CAD build for the part. Positions are in the model's coordinates, mm. A direction names the side the tool comes from. Round coordinates to 2 decimals unless told otherwise and drop trailing zeros. Order: outer loops, then holes, each group sorted by start corner. A loop starts at its lowest first (then second) coordinate and runs counter-clockwise, first axis right, second up.
```python
from build123d import *

# Parameters (mm, degrees)
CUT_EXTRUDE_START        = -3.5
SKETCH_4_R               = 17.25
SKETCH_4_R_2             = 16.25
CUT_EXTRUDE_1_DEPTH      = 0.5
HOLE_WIZARD_M2_5_2_D     = 2.05
HOLE_WIZARD_M2_5_2_DEPTH = 3.5
HOLE_WIZARD_M2_5_2_TIP   = 0.615882135
SKETCH_9_W               = 5.8
SKETCH_9_H               = 1.5
EXTRUDE_1_DEPTH          = 4
HOLE_WIZARD_M2_5_1_D     = 2.05
HOLE_WIZARD_M2_5_1_DEPTH = 3.5
HOLE_WIZARD_M2_5_1_TIP   = 0.615882135
FILLET_1_R               = 0.8
SKETCH_14_R              = 4
CUT_EXTRUDE_1_2_DEPTH    = 1.3


with BuildPart() as part:
    # 草图1 → 旋转1 (revolve)
    with BuildSketch(Plane.XY):
        Polygon((-6, 0), (-6, 1.62), (-17.25, 1.62), (-17.25, 16.62), (-3.25, 16.62), (-3.25, 0), align=None)
    revolve(axis=Axis((0, 44.719290515, 0), (0, -1, 0)))

    # 草图4 → Cut-Extrude 1 (cut)
    with BuildSketch(Plane.XZ.offset(-1.62).offset(CUT_EXTRUDE_START)):
        Circle(SKETCH_4_R)
        Circle(SKETCH_4_R_2, mode=Mode.SUBTRACT)
    extrude(amount=-CUT_EXTRUDE_1_DEPTH, mode=Mode.SUBTRACT)

    # M2.5 螺纹孔2
    with Locations(Plane(origin=(0, 1.62, 0), x_dir=(-1, 0, 0), z_dir=(0, -1, 0))):
        with Locations((-6.717514421, 6.717514421), (-6.717514421, -6.717514421), (6.717514421, -6.717514421), (6.717514421, 6.717514421)):
            Hole(HOLE_WIZARD_M2_5_2_D / 2, depth=HOLE_WIZARD_M2_5_2_DEPTH)
            with Locations((0, 0, -(HOLE_WIZARD_M2_5_2_DEPTH + HOLE_WIZARD_M2_5_2_TIP / 2))):  # 118° drill point
                Cone(0, HOLE_WIZARD_M2_5_2_D / 2, HOLE_WIZARD_M2_5_2_TIP, mode=Mode.SUBTRACT)

    # 草图9 → 凸台-拉伸1 (add)
    with BuildSketch(Plane.XZ.offset(-1.62)):
        with Locations((0, -14.5)):
            Rectangle(SKETCH_9_W, SKETCH_9_H)
    extrude(amount=EXTRUDE_1_DEPTH)

    # M2.5 螺纹孔1
    with Locations(Plane(origin=(0, 16.62, 0), x_dir=(1, 0, 0), z_dir=(0, 1, 0))):
        with Locations((-4.242640687, 4.242640687), (4.242640687, 4.242640687), (4.242640687, -4.242640687), (-4.242640687, -4.242640687)):
            Hole(HOLE_WIZARD_M2_5_1_D / 2, depth=HOLE_WIZARD_M2_5_1_DEPTH)
            with Locations((0, 0, -(HOLE_WIZARD_M2_5_1_DEPTH + HOLE_WIZARD_M2_5_1_TIP / 2))):  # 118° drill point
                Cone(0, HOLE_WIZARD_M2_5_1_D / 2, HOLE_WIZARD_M2_5_1_TIP, mode=Mode.SUBTRACT)

    # 圆角1
    fillet_1_edges = [part.edges().sort_by_distance(p)[0] for p in [
        (17.25, 16.62, 0),
    ]]
    fillet(fillet_1_edges, radius=FILLET_1_R)

    # 草图14 → Cut-Extrude 1 2 (cut)
    with BuildSketch(Plane.XZ):
        Circle(SKETCH_14_R)
    extrude(amount=-CUT_EXTRUDE_1_2_DEPTH, mode=Mode.SUBTRACT)


solid = part.part
```
1. Cut at A-A, the plane z = 0. Write the cut outline in (x, y).
2. Drill centre lines: line 1 (X direction, y = 13.5, z = 4); line 2 (X direction, y = 12.75, z = 0); line 3 (Z direction, x = -6.5, y = 2.5). Where is each one in solid material? Low to high.
3. Pin check, flat tips, straight feed: P1, Ø3, axis at y = 6.5, z = -7.5, coming from the -X side; P2, Ø1.2, axis at x = 4.24, z = 4.24, coming from the +Y side; P3, Ø1.6, axis at y = 0, z = -15, coming from the -X side. Stop position of each tip, or through.
4. Tool access for faces 5 (the face through (0, 0, -13.75)), 6 (the face through (-6.851, 3.394, -7.734)), 7 (the face through (-16.453, 3.394, -5.181)), 8 (the face through (-1.42, 0, 3.92)), 9 (the face through (5.267, 14.846, -4.288)): list every direction of +Z, -Z, +X, -X, +Y, -Y with a clear straight run to the whole face (end or side of a thin tool).
5. Mould opens along X. For faces 1 (the face through (2.579, 8.853, 1.978)), 2 (the face through (4.2, 12.6, 4.4)), 3 (the face through (13, 5.62, -10)), 4 (the face through (-16.453, 10.791, -5.181)) say: released by +X, released by -X, zero draft, split by the parting line, or undercut.
6. Cut at C-C, the plane y = -1. Write the cut outline in (x, z).
Outcome:
1. outline: (-17.25, 1.62) - (-6, 1.62) - (-6, 0) - (-4, 0) - (-4, 1.3) - (-3.25, 1.3) - (-3.25, 16.62) - (-16.45, 16.62) arc R0.8 ccw to (-17.25, 15.82) - (-17.25, 5.62) - (-16.25, 5.62) - (-16.25, 5.12) - (-17.25, 5.12) - close; (3.25, 1.3) - (4, 1.3) - (4, 0) - (6, 0) - (6, 1.62) - (17.25, 1.62) - (17.25, 5.12) - (16.25, 5.12) - (16.25, 5.62) - (17.25, 5.62) - (17.25, 15.82) arc R0.8 ccw to (16.45, 16.62) - (3.25, 16.62) - close
2. line 1: x = -16.78 to -5.24, -3.25 to 3.25, 5.24 to 16.78
2. line 2: x = -17.25 to -3.25, 3.25 to 17.25
2. line 3: z = -15.98 to -7.72, -5.72 to 5.72, 7.72 to 15.98
3. P1: stops at x = -16.17
3. P2: stops at y = 12.87
3. P3: stops at x = -2.9
4. face 5: +X, -X, -Y
4. face 6: -Y
4. face 7: +Y, -Y
4. face 8: +Z, +X, -X, -Y
4. face 9: +Y
5. face 1: undercut
5. face 2: undercut
5. face 3: zero draft
5. face 4: split by the parting line
6. outline: (-2.9, -15.25) - (2.9, -15.25) - (2.9, -13.75) - (-2.9, -13.75) - close
